Could you check a few things on this model? Use its own coordinates, in mm. A direction names the side the tool comes from. Round coordinates to 2 decimals unless told otherwise and drop trailing zeros. Write each loop counter-clockwise with the first axis right and the second up, starting at its lowest first coordinate (ties: lowest second). Pieces come first, ordered by that corner, then holes. Notation, with made-up numbers: (42, 28.5) -> (101, 28.5) arc R22 cw to (101, 40.5) -> close; hole circle Ø10 at (58, 80.5). An arc over 180 degrees is marked (long way). Answer in a Markdown table with one row per item.
from build123d import *

# Parameters (mm, degrees)
SKETCH_1_W          = 45
SKETCH_1_H          = 30
SKETCH_1_W_2        = 39
SKETCH_1_H_2        = 24
EXTRUDE_1_DEPTH     = 118
SKETCH_2_R          = 1.5
CUT_EXTRUDE_1_DEPTH = 59
SKETCH_3_W          = 31
SKETCH_3_H          = 26
CUT_EXTRUDE_2_DEPTH = 10
SKETCH_4_R          = 1.6
CUT_EXTRUDE_3_DEPTH = 50
CHAMFER_1_SIZE      = 2
FILLET_1_R          = 2
SKETCH_5_W          = 20
SKETCH_5_H          = 20
CUT_EXTRUDE_4_DEPTH = 3
SKETCH_6_R          = 1.5
CUT_EXTRUDE_5_DEPTH = 42
FILLET_2_R          = 5
SKETCH_7_R          = 1.5
CUT_EXTRUDE_6_DEPTH = 30


with BuildPart() as part:
    # 草图1 → 拉伸-薄壁1 (new body)
    with BuildSketch(Plane.XY):
        Rectangle(SKETCH_1_W, SKETCH_1_H)
        Rectangle(SKETCH_1_W_2, SKETCH_1_H_2, mode=Mode.SUBTRACT)
    extrude(amount=EXTRUDE_1_DEPTH)

    # 草图2 → 切除-拉伸1 (cut)
    with BuildSketch(Plane.ZY.offset(22.5)):
        with Locations((15.5, 8)):
            Circle(SKETCH_2_R)
        with Locations((15.5, -8)):
            Circle(SKETCH_2_R)
        with Locations((7.5, -8)):
            Circle(SKETCH_2_R)
        with Locations((7.5, 8)):
            Circle(SKETCH_2_R)
        with Locations((115, 9)):
            Circle(SKETCH_2_R)
        with Locations((97, 9)):
            Circle(SKETCH_2_R)
        with Locations((97, -9)):
            Circle(SKETCH_2_R)
        with Locations((115, -9)):
            Circle(SKETCH_2_R)
    extrude(amount=-CUT_EXTRUDE_1_DEPTH, mode=Mode.SUBTRACT)

    # 草图3 → 切除-拉伸2 (cut)
    with BuildSketch(Plane(origin=(0, -12, 0), x_dir=(1, 0, 0), z_dir=(0, 1, 0))):
        with Locations((0, -13)):
            Rectangle(SKETCH_3_W, SKETCH_3_H)
    extrude(amount=-CUT_EXTRUDE_2_DEPTH, mode=Mode.SUBTRACT)

    # 草图4 → 切除-拉伸3 (cut)
    with BuildSketch(Plane(origin=(22.5, 0, 0), x_dir=(0, 0, -1), z_dir=(1, 0, 0))):
        with Locations((-25.5, 5)):
            Circle(SKETCH_4_R)
        with Locations((-45.5, 5)):
            Circle(SKETCH_4_R)
        with Locations((-65.5, 5)):
            Circle(SKETCH_4_R)
        with Locations((-85.5, 5)):
            Circle(SKETCH_4_R)
        with Locations((-105.5, 5)):
            Circle(SKETCH_4_R)
    extrude(amount=-CUT_EXTRUDE_3_DEPTH, mode=Mode.SUBTRACT)

    # 倒角1
    chamfer_1_edges = [part.edges().sort_by_distance(p)[0] for p in [
        (22.5, 9, 95.5),
        (-22.5, 9, 95.5),
        (22.5, -9, 95.5),
        (-22.5, -9, 95.5),
    ]]
    chamfer(chamfer_1_edges, length=CHAMFER_1_SIZE)

    # 圆角1
    fillet_1_edges = [part.edges().sort_by_distance(p)[0] for p in [
        (15.5, -13.5, 0),
        (15.5, -13.5, 26),
        (-15.5, -13.5, 26),
        (-15.5, -13.5, 0),
    ]]
    fillet(fillet_1_edges, radius=FILLET_1_R)

    # 草图5 → 切除-拉伸4 (cut)
    with BuildSketch(Plane(origin=(0, 15, 0), x_dir=(1, 0, 0), z_dir=(0, 1, 0))):
        with Locations((0, -93)):
            Rectangle(SKETCH_5_W, SKETCH_5_H)
    extrude(amount=-CUT_EXTRUDE_4_DEPTH, mode=Mode.SUBTRACT)

    # 草图6 → 切除-拉伸5 (cut)
    with BuildSketch(Plane(origin=(0, 15, 0), x_dir=(1, 0, 0), z_dir=(0, 1, 0))):
        with Locations(Location((10, -73, 0), (0, 0, 270))):
            Circle(SKETCH_6_R)
        with Locations(Location((-10, -73, 0), (0, 0, 270))):
            Circle(SKETCH_6_R)
        with Locations(Location((-10, -53, 0), (0, 0, 270))):
            Circle(SKETCH_6_R)
        with Locations(Location((10, -53, 0), (0, 0, 270))):
            Circle(SKETCH_6_R)
        with Locations(Location((-10, -33, 0), (0, 0, 270))):
            Circle(SKETCH_6_R)
        with Locations(Location((10, -33, 0), (0, 0, 270))):
            Circle(SKETCH_6_R)
        with Locations(Location((-10, -13, 0), (0, 0, 270))):
            Circle(SKETCH_6_R)
        with Locations(Location((10, -13, 0), (0, 0, 270))):
            Circle(SKETCH_6_R)
    extrude(amount=-CUT_EXTRUDE_5_DEPTH, mode=Mode.SUBTRACT)

    # 圆角2
    fillet_2_edges = [part.edges().sort_by_distance(p)[0] for p in [
        (10, 13.5, 83),
        (10, 13.5, 103),
        (-10, 13.5, 103),
        (-10, 13.5, 83),
    ]]
    fillet(fillet_2_edges, radius=FILLET_2_R)

    # 草图7 → 切除-拉伸6 (cut)
    with BuildSketch(Plane(origin=(0, 15, 0), x_dir=(1, 0, 0), z_dir=(0, 1, 0))):
        with Locations(Location((8, -114.5, 0), (0, 0, 270))):
            Circle(SKETCH_7_R)
        with Locations(Location((-8, -114.5, 0), (0, 0, 270))):
            Circle(SKETCH_7_R)
    extrude(amount=-CUT_EXTRUDE_6_DEPTH, mode=Mode.SUBTRACT)


solid = part.part
1) Imagine slicing it at D-D, the plane z = 18.5. Please give me the cut outline in (x, y), plus the area to 3 significant figures.
Findings:
| item | result |
|---|---|
| outline | (-22.5, -15) -> (-15.5, -15) -> (-15.5, -12) -> (-19.5, -12) -> (-19.5, 12) -> (19.5, 12) -> (19.5, -12) -> (15.5, -12) -> (15.5, -15) -> (22.5, -15) -> (22.5, 15) -> (-22.5, 15) -> close |
| area | 321 mm^2 |
2) Imagine slicing it at A-A, the plane z = 53. Please give me the cut outline in (x, y).
Findings:
| item | result |
|---|---|
| outline | (-22.5, -15) -> (-11.5, -15) -> (-11.5, -12) -> (-19.5, -12) -> (-19.5, 12) -> (-11.5, 12) -> (-11.5, 15) -> (-22.5, 15) -> close; (-8.5, -15) -> (8.5, -15) -> (8.5, -12) -> (-8.5, -12) -> close; (-8.5, 12) -> (8.5, 12) -> (8.5, 15) -> (-8.5, 15) -> close; (11.5, -15) -> (22.5, -15) -> (22.5, 15) -> (11.5, 15) -> (11.5, 12) -> (19.5, 12) -> (19.5, -12) -> (11.5, -12) -> close |
3) Please list where these lines run through material, in increasing order: line 1 (Y direction, x = -21.3, z = 15.5); line 2 (X direction, y = -12.8, z = 73); line 3 (Y direction, x = -13, z = 97.5).
Findings:
| item | result |
|---|---|
| line 1 | y = -15 to -9.5, -6.5 to 6.5, 9.5 to 15 |
| line 2 | x = -22.5 to -11.5, -8.5 to 8.5, 11.5 to 22.5 |
| line 3 | y = -15 to -12, 12 to 15 |
4) Imagine slicing it at B-B, the plane z = 65. Please give me the cut outline in (x, y).
Findings:
| item | result |
|---|---|
| outline | (-22.5, -15) -> (22.5, -15) -> (22.5, 3.48) -> (19.5, 3.48) -> (19.5, -12) -> (-19.5, -12) -> (-19.5, 3.48) -> (-22.5, 3.48) -> close; (-22.5, 6.52) -> (-19.5, 6.52) -> (-19.5, 12) -> (19.5, 12) -> (19.5, 6.52) -> (22.5, 6.52) -> (22.5, 15) -> (-22.5, 15) -> close |
5) Thinking about a two-plate mould opening in Z: for faces 4 (the face through (-21, -9, 99)), 5 (the face through (-19.5, 0, 58)), 6 (the face through (-20.98, 3.58, 24.76)), 7 (the face through (-14.93, -13.52, 25.4)), which applies, +Z half, -Z half, draft (parallel to the pull), parting line (faces both ways), or undercut?
Findings:
| item | result |
|---|---|
| face 4 | undercut |
| face 5 | draft |
| face 6 | undercut |
| face 7 | -Z half |
6) Imagine slicing it at C-C, the plane z = 85.5. Please give me the cut outline in (x, y), plus the area to 3 significant figures.
Findings:
| item | result |
|---|---|
| outline | (-22.5, -15) -> (22.5, -15) -> (22.5, 3.4) -> (19.5, 3.4) -> (19.5, -12) -> (-19.5, -12) -> (-19.5, 3.4) -> (-22.5, 3.4) -> close; (-22.5, 6.6) -> (-19.5, 6.6) -> (-19.5, 12) -> (-9.33, 12) -> (-9.33, 15) -> (-22.5, 15) -> close; (9.33, 12) -> (19.5, 12) -> (19.5, 6.6) -> (22.5, 6.6) -> (22.5, 15) -> (9.33, 15) -> close |
| area | 339 mm^2 |
7) For pin 1 (2.5 mm diameter, centred on y = -9, z = 97, fed in from +X); pin 2 (3.5 mm diameter, centred on x = 0.5, y = -13, fed in from -Z), each with a flat end and sliding along its axis, tell me the tip position at first contact or that it passes through.
Findings:
| item | result |
|---|---|
| pin 1 | passes through |
| pin 2 | stops at z = 26 |
8) For faces 1 (the face through (15.5, -13, 13)), 2 (the face through (-9, 13, 85)), 3 (the face through (0, -12, 71)), which set-ups out of +Z, -Z, +X, -X, +Y, -Y let a thin tool reach every point of the face, with its end or its side?
Findings:
| item | result |
|---|---|
| face 1 | -Z, -Y |
| face 2 | +Y |
| face 3 | +Z, -Z |
